Can you work these out from the model? Positions are in its coordinate system, mm. A direction names the side the tool comes from. Coordinates: 2 decimals unless noted, no trailing zeros. Order: outer loops, then holes, each group sorted by start corner. A loop starts at its lowest first (then second) coordinate and runs counter-clockwise, first axis right, second up. Notation, with made-up numbers: (25.25, 74.5) -> (29.25, 74.5) arc R27 ccw to (29.25, 107.5) -> close; hole circle Ø5 at (-24.75, -1). An arc over 180 degrees is marked (long way). Write item = value, one per line.
Autodesk Inventor part; units mm, degrees
ref_plane "YZ Plane" through (0, 0, 0) normal (1, 0, 0) x (0, 1, 0)
ref_plane "XZ Plane" through (0, 0, 0) normal (0, 1, 0) x (-1, 0, 0)
ref_plane "XY Plane" through (0, 0, 0) normal (0, 0, 1) x (1, 0, 0)
sketch "Sketch1" plane through (0, 0, 0) normal (1, 0, 0) x (0, 1, 0)
  circle A0 centre (0, 0) radius 4
  circle A1 centre (0, 0) radius 17.5
  dimension "d0" = 8
  dimension "d1" = 35
extrude "Extrusion1" add sketch "Sketch1" along normal blind 20
chamfer "Chamfer1" distance 2 angle 45 2 edges at (0, -17.5, 0) (20, -17.5, 0)
sketch "Sketch2" plane through (0, 0, 0) normal (0, 1, 0) x (-1, 0, 0)
  line L0 (0, 0) -> (-10, 0)
  circle A0 centre (-10, 0) radius 2.5
  dimension "d7" = 10
  dimension "d8" = 5
extrude "Extrusion2" cut sketch "Sketch2" against normal blind 20
thread "Thread1"
properties part number "counterweight#" material "Stainless Steel"
Item 1: I'm going to push flat-ended pins straight in: P1, Ø12, axis at x = 8, y = -12.5, coming from the -Z side; P2, Ø3, axis at x = 5, y = -13, coming from the +Z side; P3, Ø3, axis at x = 5, z = 2.5, coming from the +Y side; P4, Ø7, axis at y = 0, z = 0, coming from the -X side. Where does each tip first touch, or does it pass through?
A:
P1 = -16.25
P2 = 13.19
P3 = 17.47
P4 = through
Item 2: If I drill on probe 1 along Y at (x, z) = (6.5, 0); probe 2 along Y at (x, z) = (4, -2), over which ranges is the centre line in solid material (lowest first)?
A:
probe_1 = -17.5 to -4, 4 to 17.5
probe_2 = -17.39 to -3.46, 3.46 to 17.39
Item 3: I want a section at B-B, the plane z = 0. Please give me the cut outline in (x, y), plus the area to 4 significant figures.
A:
outline = (0, -15.5) -> (2, -17.5) -> (7.5, -17.5) -> (7.5, -4) -> (0, -4) -> close; (0, 4) -> (20, 4) -> (20, 15.5) -> (18, 17.5) -> (2, 17.5) -> (0, 15.5) -> close; (12.5, -17.5) -> (18, -17.5) -> (20, -15.5) -> (20, -4) -> (12.5, -4) -> close
area = 464.5 mm2
Item 4: I want a section at C-C, the plane x = 4.75. Please give me the cut outline in (y, z).
A:
outline = circle Ø35 at (0, 0); hole circle Ø8 at (0, 0)
Item 5: I want a section at D-D, the plane x = 8.5. Please give me the cut outline in (y, z), plus the area to 3 significant figures.
A:
outline = (-17.39, -2) arc R17.5 ccw (long way) to (-17.39, 2) -> (-3.46, 2) arc R4 cw (long way) to (-3.46, -2) -> close
area = 857 mm2
Item 6: If we mould it in two halves opening along Y, with no side actions, what happens to faces 3 (the conical face through (0.125, -3.387, -15.254)), 4 (the flat face through (20, 3, -3)), 5 (the cylindrical face through (9.86, 3.815, -1.201))? For each: pulls with the +Y half, pulls with the -Y half, needs draft (parallel to the pull), parting line crosses it, or undercut.
A:
face_3 = parting line crosses it
face_4 = needs draft
face_5 = undercut
Item 7: I want a section at A-A, the plane y = 0. Please give me the cut outline in (x, z).
A:
outline = (0, -15.5) -> (2, -17.5) -> (18, -17.5) -> (20, -15.5) -> (20, -4) -> (0, -4) -> close; (0, 4) -> (20, 4) -> (20, 15.5) -> (18, 17.5) -> (2, 17.5) -> (0, 15.5) -> close
Item 8: For faces 1 (the cylindrical face through (9.888, 16.166, 6.703)), 2 (the cylindrical face through (12.5, -10.2, 0.1)), which set-ups out of +Z, -Z, +X, -X, +Y, -Y let a thin tool reach every point of the face, with its end or its side?
A:
face_1 = +X, -X
face_2 = -Y
